from build123d import *

# Parameters (mm, degrees)
SKETCH2_R           = 32.183564388
BOSS_EXTRUDE1_DEPTH = 7
SKETCH3_R           = 10
CUT_EXTRUDE1_DEPTH  = 47.049577994


with BuildPart() as part:
    # Sketch2 → Boss-Extrude1 (new body)
    with BuildSketch(Plane.XY):
        Circle(SKETCH2_R)
    extrude(amount=BOSS_EXTRUDE1_DEPTH)

    # Sketch3 → Cut-Extrude1 (cut, through all)
    with BuildSketch(Plane.XY.offset(7)):
        Circle(SKETCH3_R)
    extrude(amount=-CUT_EXTRUDE1_DEPTH, mode=Mode.SUBTRACT)

    # Sketch4 → Cut-Revolve1 (revolve, cut)
    with BuildSketch(Plane(origin=(0, 0, 0), x_dir=(1, 0, 0), z_dir=(0, 1, 0))):
        with BuildLine():
            Line((-22.244858179, -7), (0, -7))
            Line((0, -7), (0, 4.212792064))
            Line((0, 4.212792064), (-10, 4.212792064))
            ThreePointArc((-10, 4.212792064), (-17.06939941, -0.359471059), (-22.244858179, -7))
        make_face()
    revolve(axis=Axis((0, 0, -16.764248705), (0, 0, 1)), mode=Mode.SUBTRACT)


solid = part.part
Here's how the part is built. I have some questions about the finished solid (model axes, mm). Round coordinates to 2 decimals unless told otherwise and drop trailing zeros. Loops run counter-clockwise (first coordinate to the right, second up) from the corner with the lowest first, then second, coordinate; pieces in that order, holes last.
1. If I drill on line 1 along Y through (x, z) = (-14, 2.75); line 2 along X through (y, z) = (2, 6); line 3 along X through (y, z) = (3.5, 6.5), over which ranges is the centre line in solid material (lowest first)?
Answer list:
line 1: y = -28.98 to -13.37, 13.37 to 28.98
line 2: x = -32.12 to -21.58, 21.58 to 32.12
line 3: x = -31.99 to -21.69, 21.69 to 31.99
2. For P1, Ø2, axis at x = 1, y = -17.5, coming from the +Z side; P2, Ø3, axis at x = -1, z = 3, coming from the +Y side; P3, Ø3, axis at y = -18, z = 6, coming from the -X side, each with a flat end and sliding along its axis, tell me the tip position at first contact or that it passes through.
Answer list:
P1: stops at z = 1.81
P2: stops at y = 32.18
P3: stops at x = -27.63
3. If we section it at C-C on z = 1.25: Write out the boundary of the cut face in (x, y).
Answer list:
outline: circle Ø64.37 at (0, 0); hole circle Ø35.99 at (0, 0)
4. If we section it at A-A on y = 14.5: Write out the boundary of the cut face in (x, z).
Answer list:
outline: (-28.73, 0) - (-8.22, 0) arc R20.7 cw to (-16.87, 7) - (-28.73, 7) - close; (8.22, 0) - (28.73, 0) - (28.73, 7) - (16.87, 7) arc R20.7 cw to start
5. If we section it at D-D on y = 24: Write out the boundary of the cut face in (x, z), plus the area to 3 significant figures.
Answer list:
outline: (-21.44, 0) - (21.44, 0) - (21.44, 7) - (-21.44, 7) - close
area: 300 mm2
6. If we section it at B-B on x = -15.5: Write out the boundary of the cut face in (y, z), plus the area to 3 significant figures.
Answer list:
outline: (-28.21, 0) - (-6.13, 0) arc R19.96 cw to (-15.96, 7) - (-28.21, 7) - close; (6.13, 0) - (28.21, 0) - (28.21, 7) - (15.96, 7) arc R19.96 cw to start
area: 225 mm2
